from build123d import *

# Parameters (mm, degrees)
F0_R     = 19.05
F0_R_2   = 1.5875
F1_DEPTH = 6.35
F3_D     = 6.35


with BuildPart() as f1:
    # F0 (on Top) → F1 (new body)
    with BuildSketch(Plane.XY):
        with Locations((-3.877292, -5.028827)):
            Circle(F0_R)
        with Locations((-6.599113, -3.81)):
            Circle(F0_R_2, mode=Mode.SUBTRACT)
        with Locations((6.599114, -3.809999)):
            Circle(F0_R_2, mode=Mode.SUBTRACT)
        with Locations((0, 7.62)):
            Circle(F0_R_2, mode=Mode.SUBTRACT)
    extrude(amount=F1_DEPTH)

    # F3 (through all)
    with Locations(Plane.XY.offset(6.35)):
        with Locations((0, 0)):
            Hole(F3_D / 2)


solid = f1.part
Can you work these out from the model? Positions are in its coordinate system, mm. Give positions to 0.01 mm unless a question says otherwise; leave off trailing zeros. Loops run counter-clockwise (first coordinate to the right, second up) from the corner with the lowest first, then second, coordinate; pieces in that order, holes last. Notation, with made-up numbers: M 67,-15.75 L 117,-15.75 A19 cw 117,-4.75 Z; hole C -29.75,59.5 d6. An arc over 180 degrees is marked long. One line per item, written item: value. Start each with the question number.
1) If we section it at B-B, the plane y = 0: Write out the boundary of the cut face in (x, z) (3 decimals).
2) If we section it at D-D, the plane y = 7.62: Write out the boundary of the cut face in (x, z), and give its area (3 significant figures).
3) If we section it at A-A, the plane x = 0: Give the number of separate pieces and of enclosed holes in the cut face, and give its area (3 significant figures).
4) I'm going to push flat-ended pins straight in: pin 1 (3 mm diameter, centred on x = -5.5, z = 1.5, fed in from -Y); pin 2 (1.5 mm diameter, centred on x = -7, z = 4.5, fed in from +Y). Where does each tip first touch, or does it pass through?
5) Thinking about a two-plate mould opening in Y: for faces 1 (the face through (-8.185, -3.74, 3.131)), 2 (the face through (14.293, 0.693, 3.131)), 3 (the face through (-0.34, 6.07, 3.13)), 4 (the face through (-4, -5, 0)), which applies, +Y half, -Y half, draft (parallel to the pull), parting line (faces both ways), or undercut?
6) If I drill on line 1 (X direction, y = -4, z = 6); line 2 (Y direction, x = 0, z = 5) (1 decimal); line 3 (X direction, y = 2.5, z = 6.25), over which ranges is the centre line in solid material (lowest first)? Write a range as [from, to].
Completed:
1. outline: M -22.252,0 L -3.175,0 L -3.175,6.35 L -22.252,6.35 Z; M 3.175,0 L 14.497,0 L 14.497,6.35 L 3.175,6.35 Z
2. outline: M -18.12,0 L -1.59,0 L -1.59,6.35 L -18.12,6.35 Z; M 1.59,0 L 10.37,0 L 10.37,6.35 L 1.59,6.35 Z
2. area: 161 mm^2
3. separate pieces: 3
3. enclosed holes: 0
3. area: 176 mm^2
4. pin 1: stops at y = -24.08
4. pin 2: stops at y = 13.87
5. face 1: undercut
5. face 2: parting line
5. face 3: undercut
5. face 4: draft
6. line 1: x = [-22.9, -8.18], [-5.02, 5.02], [8.18, 15.14]
6. line 2: y = [-23.7, -3.2], [3.2, 6], [9.2, 13.6]
6. line 3: x = [-21.38, -1.96], [1.96, 13.62]
